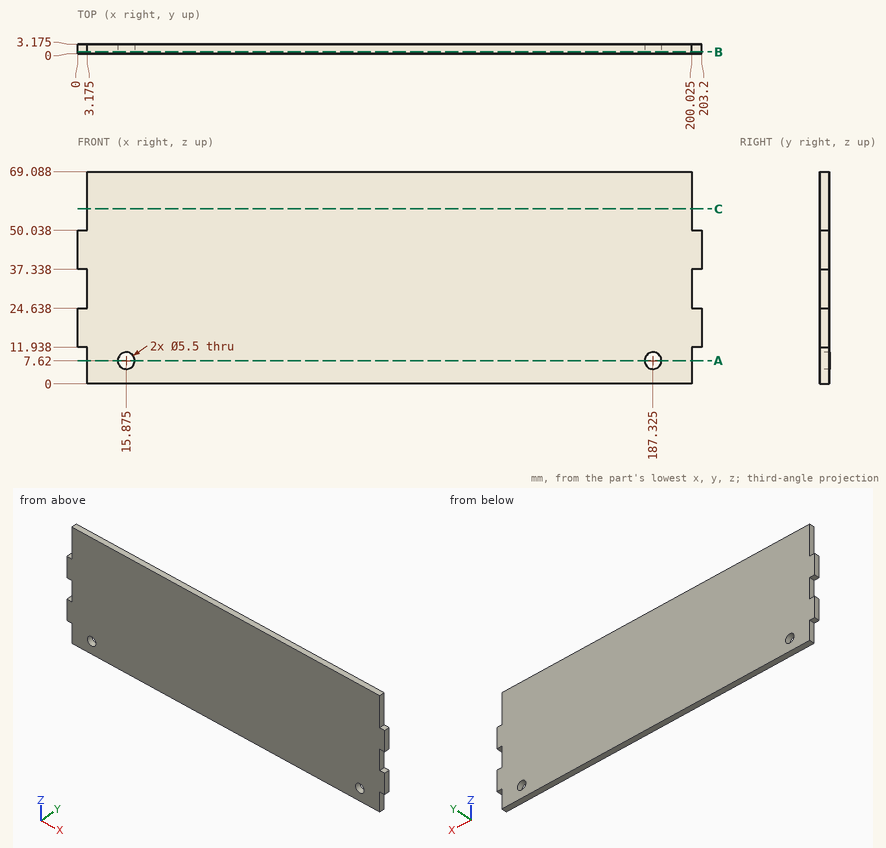
Verification items for this drawing (mm, ordinates from the low corner). Give positions to 0.01 mm unless a question says otherwise; leave off trailing zeros. Loops run counter-clockwise (first coordinate to the right, second up) from the corner with the lowest first, then second, coordinate; pieces in that order, holes last. Notation, with made-up numbers: M 89.5,-21 L 125.5,-21 A8 cw 125.5,-8 Z; hole C 18.25,84 d9. An arc over 180 degrees is marked long. Answer in a Markdown table with one row per item.
1) Cross-section at B-B (y = 0.6). Enter the section's corners in (x, z) (3 decimals).
Solutions:
| item | result |
|---|---|
| outline | M 0,11.938 L 3.175,11.938 L 3.175,0 L 200.025,0 L 200.025,11.938 L 203.2,11.938 L 203.2,24.638 L 200.025,24.638 L 200.025,37.338 L 203.2,37.338 L 203.2,50.038 L 200.025,50.038 L 200.025,69.088 L 3.175,69.088 L 3.175,50.038 L 0,50.038 L 0,37.338 L 3.175,37.338 L 3.175,24.638 L 0,24.638 Z; hole C 15.875,7.62 d5.5; hole C 187.325,7.62 d5.5 |
2) Depth check by flat-ended pin: pin 1 (1.6 mm diameter, centred on x = 201.5, y = 2, fed in from +Z); pin 2 (1 mm diameter, centred on y = 2, z = 56, fed in from +X) (3 decimals); pin 3 (1.5 mm diameter, centred on x = 24, y = 1.5, fed in from -Z); pin 4 (1 mm diameter, centred on x = 1.5, y = 2, fed in from -Z). Enter the tip coordinate at first touch or a pass-through.
Solutions:
| item | result |
|---|---|
| pin 1 | stops at z = 50.04 |
| pin 2 | stops at x = 200.025 |
| pin 3 | stops at z = 0 |
| pin 4 | stops at z = 11.94 |
3) Cross-section at A-A (z = 7.62). Enter the section's corners in (x, y) (3 decimals), plus the area to 3 significant figures.
Solutions:
| item | result |
|---|---|
| outline | M 3.175,0 L 13.125,0 L 13.125,3.175 L 3.175,3.175 Z; M 18.625,0 L 184.575,0 L 184.575,3.175 L 18.625,3.175 Z; M 190.075,0 L 200.025,0 L 200.025,3.175 L 190.075,3.175 Z |
| area | 590 mm^2 |
4) Thickness scan on line 1 (X direction, y = 1.95, z = 7.62) (3 decimals); line 2 (X direction, y = 2.25, z = 26.5) (3 decimals); line 3 (X direction, y = 2.2, z = 9.5) (3 decimals). Record the ranges inside material, lowest first.
Solutions:
| item | result |
|---|---|
| line 1 | x = 3.175 to 13.125, 18.625 to 184.575, 190.075 to 200.025 |
| line 2 | x = 3.175 to 200.025 |
| line 3 | x = 3.175 to 13.868, 17.882 to 185.318, 189.332 to 200.025 |
5) Cross-section at C-C (z = 57). Enter the section's corners in (x, y) (3 decimals).
Solutions:
| item | result |
|---|---|
| outline | M 3.175,0 L 200.025,0 L 200.025,3.175 L 3.175,3.175 Z |
